Autodesk Inventor part; units mm, degrees
ref_plane "YZ Plane" through (0, 0, 0) normal (1, 0, 0) x (0, 1, 0)
ref_plane "XZ Plane" through (0, 0, 0) normal (0, 1, 0) x (-1, 0, 0)
ref_plane "XY Plane" through (0, 0, 0) normal (0, 0, 1) x (1, 0, 0)
sketch "Sketch1" plane through (0, 0, 0) normal (0, 1, 0) x (-1, 0, 0)
  line L0 (11.1299, 50.0199) -> (11.1299, 62.0199)
  line L1 (-17.8701, 62.0199) -> (-17.8701, 50.0199)
  line L2 (-17.8701, 50.0199) -> (-3.3701, 50.0199)
  line L3 (-3.3701, 50.0199) -> (-3.3701, 62.0199) construction
  line L4 (-17.8701, 56.0199) -> (-3.3701, 56.0199) construction
  line L5 (-17.8701, 62.0199) -> (11.1299, 62.0199)
  line L6 (-17.8701, 62.0199) -> (-8.8701, 62.0199)
  line L7 (-8.8701, 62.0199) -> (-8.8701, 68.0199)
  line L8 (-8.8701, 68.0199) -> (-17.8701, 68.0199)
  line L9 (-17.8701, 68.0199) -> (-17.8701, 62.0199)
  line L10 (11.1299, 62.0199) -> (2.1299, 62.0199)
  line L11 (2.1299, 62.0199) -> (2.1299, 68.0199)
  line L12 (2.1299, 68.0199) -> (11.1299, 68.0199)
  line L13 (11.1299, 68.0199) -> (11.1299, 62.0199)
  line L14 (-3.3701, 56.0199) -> (11.1299, 56.0199) construction
  line L15 (-3.3701, 50.0199) -> (11.1299, 50.0199)
  line L16 (-0.3701, 59.0199) -> (8.6299, 59.0199)
  line L17 (8.6299, 59.0199) -> (8.6299, 53.0199)
  line L18 (8.6299, 53.0199) -> (-0.3701, 53.0199)
  line L19 (-0.3701, 53.0199) -> (-0.3701, 59.0199)
  line L20 (-0.3701, 59.0199) -> (8.6299, 53.0199) construction
  line L21 (8.6299, 59.0199) -> (-0.3701, 53.0199) construction
  line L22 (-6.3701, 59.0199) -> (-15.3701, 59.0199)
  line L23 (-15.3701, 59.0199) -> (-15.3701, 53.0199)
  line L24 (-15.3701, 53.0199) -> (-6.3701, 53.0199)
  line L25 (-6.3701, 53.0199) -> (-6.3701, 59.0199)
  line L26 (-6.3701, 59.0199) -> (-15.3701, 53.0199) construction
  line L27 (-15.3701, 59.0199) -> (-6.3701, 53.0199) construction
  line L28 (11.1299, 50.0199) -> (14.1299, 50.0199)
  line L29 (14.1299, 50.0199) -> (14.1299, 62.0199)
  line L30 (14.1299, 62.0199) -> (11.1299, 62.0199)
  line L31 (11.1299, 62.0199) -> (11.1299, 50.0199)
  line L32 (-17.8701, 50.0199) -> (-17.8701, 62.0199)
  line L33 (-17.8701, 50.0199) -> (-20.8701, 50.0199)
  line L34 (-20.8701, 50.0199) -> (-20.8701, 62.0199)
  line L35 (-20.8701, 62.0199) -> (-17.8701, 62.0199)
  line L36 (-17.8701, 62.0199) -> (-17.8701, 50.0199)
  point P0 (4.1299, 56.0199)
  point P1 (-10.8701, 56.0199)
  dimension "d0" = 29
  dimension "d1" = 12
  dimension "d18" = 9
  dimension "d19" = 6
  dimension "d20" = 14.5
  dimension "d61" = 9
  dimension "d62" = 6
  dimension "d63" = 6
  dimension "d64" = 3
  dimension "d65" = 3
  dimension "d66" = 12
extrude "Extrusion1" add sketch "Sketch1" along normal blind 6
equation "\"d66\" = d1"
properties part number "thumper-bumper-sidewall2-v3"
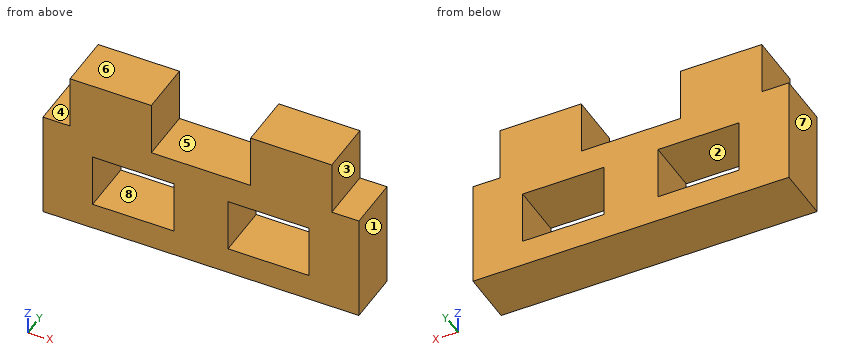
Geometry: final body of the model. Coordinates: model frame, mm. Face numbers are marked on the shaded views. A direction names the side the tool comes from. Coordinates: 2 decimals unless noted, no trailing zeros. Loops run counter-clockwise (first coordinate to the right, second up) from the corner with the lowest first, then second, coordinate; pieces in that order, holes last. Notation, with made-up numbers: (42, -2.5) - (49, -2.5) arc R29 ccw to (49, 31.5) - close; hole circle Ø1 at (17.25, -10.75). An arc over 180 degrees is marked (long way). Put each result on its own line as item: value. Start each with the question number.
Q1. Pin query (flat end, axial travel): pin 1 Ø1 at (y, z) = (4.5, 63) entering from +X; pin 2 Ø0.9 at (x, y) = (19, 4) entering from +Z; pin 3 Ø1.8 at (y, z) = (2, 64) entering from -X. Return the tip coordinate at first contact, or that it passes through.
Q2. Cut plane B-B, the plane y = 1.7. Return loops of the section in (x, z).
Q3. Cut plane D-D, the plane z = 63.25. Return loops of the section in (x, y), and give its area (3 significant figures).
Q4. Cut plane C-C, the plane x = -0.5. Return loops of the section in (y, z).
Q5. Set-up query: the marked faces 1, 2, 3, 4 and 5. Return all of +Z, -Z, +X, -X, +Y, -Y with unobstructed straight access to the full face (end or side cutting, diameter ignored); none if empty.
Q6. Cut plane A-A, the plane z = 54. Return loops of the section in (x, y), and give its area (3 significant figures).
Q7. Line query: line 1 (X direction, y = 0.35, z = 53.25); line 2 (X direction, y = 4.75, z = 66); line 3 (Z direction, x = 7.5, y = 1.5). Output: solid intervals per line, ascending.
Q8. Pull-direction query (Z, two-part tool) for the marked faces 6, 7 and 8; classes: released by +Z, released by -Z, zero draft, split by the parting line, or undercut.
Filled sheet:
1. pin 1: x = 17.87
1. pin 2: z = 62.02
1. pin 3: x = -11.13
2. outline: (-14.13, 50.02) - (20.87, 50.02) - (20.87, 62.02) - (17.87, 62.02) - (17.87, 68.02) - (8.87, 68.02) - (8.87, 62.02) - (-2.13, 62.02) - (-2.13, 68.02) - (-11.13, 68.02) - (-11.13, 62.02) - (-14.13, 62.02) - close; hole (-8.63, 53.02) - (0.37, 53.02) - (0.37, 59.02) - (-8.63, 59.02) - close; hole (6.37, 53.02) - (15.37, 53.02) - (15.37, 59.02) - (6.37, 59.02) - close
3. outline: (-11.13, 0) - (-2.13, 0) - (-2.13, 6) - (-11.13, 6) - close; (8.87, 0) - (17.87, 0) - (17.87, 6) - (8.87, 6) - close
3. area: 108 mm²
4. outline: (0, 50.02) - (6, 50.02) - (6, 53.02) - (0, 53.02) - close; (0, 59.02) - (6, 59.02) - (6, 62.02) - (0, 62.02) - close
5. face 1: +Z, -Z, +X, +Y, -Y
5. face 2: +Y, -Y
5. face 3: +Z, +X, +Y, -Y
5. face 4: +Z, -X, +Y, -Y
5. face 5: +Z, +Y, -Y
6. outline: (-14.13, 0) - (-8.63, 0) - (-8.63, 6) - (-14.13, 6) - close; (0.37, 0) - (6.37, 0) - (6.37, 6) - (0.37, 6) - close; (15.37, 0) - (20.87, 0) - (20.87, 6) - (15.37, 6) - close
6. area: 102 mm²
7. line 1: -14.13 to -8.63, 0.37 to 6.37, 15.37 to 20.87
7. line 2: -11.13 to -2.13, 8.87 to 17.87
7. line 3: 50.02 to 53.02, 59.02 to 62.02
8. face 6: released by +Z
8. face 7: zero draft
8. face 8: undercut
